from build123d import *

# Parameters (mm, degrees)
F0_W     = 347
F0_H     = 3
F0_W_2   = 3
F0_H_2   = 247
F1_DEPTH = 60


with BuildPart() as f1:
    # F0 (on Front) → F1 (new body, symmetric)
    with BuildSketch(Plane.XZ):
        with Locations((-176.5, 1.5)):
            Rectangle(F0_W, F0_H)
        with Locations((-1.5, 1.5)):
            Rectangle(F0_W_2, F0_H)
        with Locations((-1.5, 126.5)):
            Rectangle(F0_W_2, F0_H_2)
    extrude(amount=F1_DEPTH, both=True)


solid = f1.part
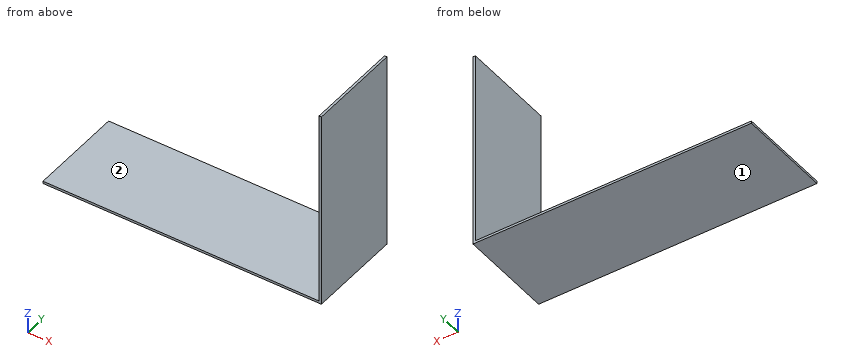
Build history of the part. All positions in model axes, mm. Face numbers are marked on the shaded views. A direction names the side the tool comes from. Round coordinates to 2 decimals unless told otherwise and drop trailing zeros. Write each loop counter-clockwise with the first axis right and the second up, starting at its lowest first coordinate (ties: lowest second). Pieces come first, ordered by that corner, then holes. Notation, with made-up numbers: (34.25, 8.5) - (65.25, 8.5) arc R25 cw to (65.25, 31.5) - close; hole circle Ø3 at (24.25, -39). An arc over 180 degrees is marked (long way). One line per question, with ' | ' between items.
1. Band-saw the part on C-C, the plane z = 64. Write the cut outline in (x, y), and give its area (3 significant figures).
Results are:
outline: (-3, -60) - (0, -60) - (0, 60) - (-3, 60) - close | area: 360 mm^2
2. Band-saw the part on A-A, the plane y = -33. Write the cut outline in (x, z), and give its area (3 significant figures).
Results are:
outline: (-350, 0) - (0, 0) - (0, 250) - (-3, 250) - (-3, 3) - (-350, 3) - close | area: 1,790 mm^2
3. Drill centre lines: line 1 along X through (y, z) = (20, 53); line 2 along Z through (x, y) = (-250, 54). Where is each one in solid material? Low to high. Write a range as from..to.
Results are:
line 1: -3..0 | line 2: 0..3
4. Drop flat-ended pins along their axis: pin 1 Ø5 at (x, y) = (-134.5, 7.5) entering from +Z; pin 2 Ø2 at (y, z) = (9.5, 212.5) entering from -X. Give the stop position or say it passes through.
Results are:
pin 1: z = 3 | pin 2: x = -3
5. Band-saw the part on B-B, the plane x = -82. Write the cut outline in (y, z).
Results are:
outline: (-60, 0) - (60, 0) - (60, 3) - (-60, 3) - close
6. Tool access for the marked faces 1 and 2: list every direction of +Z, -Z, +X, -X, +Y, -Y with a clear straight run to the whole face (end or side of a thin tool).
Results are:
face 1: -Z, +X, -X, +Y, -Y | face 2: +Z, -X, +Y, -Y
